Here's how the part is built. I have some questions about the finished solid (model axes, mm). Face numbers are marked on the shaded views. Coordinates: 2 decimals unless noted, no trailing zeros. Write each loop counter-clockwise with the first axis right and the second up, starting at its lowest first coordinate (ties: lowest second). Pieces come first, ordered by that corner, then holes.
Item 1: I want a section at D-D (x = 6.5). Please give me the cut outline in (y, z).
Item 2: I want a section at B-B (z = 1). Please give me the cut outline in (x, y), and give its area (3 significant figures).
Item 3: I'm going to push flat-ended pins straight in: P1, Ø6.5, axis at y = 54.3, z = 7.5, coming from the -X side; P2, Ø7.5, axis at y = 50, z = 11, coming from the +X side; P3, Ø1.5, axis at x = 2, z = 10.5, coming from the +Y side; P4, Ø5, axis at x = -1, z = 9, coming from the -Y side. Where does each tip first touch, or does it pass through?
Item 4: I want a section at C-C (y = 37). Please give me the cut outline in (x, z), and give its area (3 significant figures).
Item 5: If we mould it in two halves opening along X, with no side actions, what happens to the marked faces 1, 2, 3 and 4? For each: pulls with the +X half, pulls with the -X half, needs draft (parallel to the pull), parting line crosses it, or undercut.
Item 6: I want a section at A-A (y = 2). Please give me the cut outline in (x, z), and give its area (3 significant figures).
Item 7: Please list where these lines run through material, in increasing order: line 1 (X direction, y = 49, z = 6.25); line 2 (X direction, y = 21, z = 7.5); line 3 (Y direction, x = -5.75, z = 5.75).
from build123d import *

# Parameters (mm, degrees)
F1_DEPTH       = 15
F3_D           = 5.2
F3_DEPTH       = 30
F3_CBORE_D     = 10.2
F3_CBORE_DEPTH = 5
F3_TIP         = 1.5622376095
F4_W           = 8.2
F4_H           = 4.3
F5_DEPTH       = 12.4
F6_R           = 4.1
F7_DEPTH       = 25
F8_R           = 7.5
F9_R           = 7.5
F10_R          = 7.49999
F11_SIZE       = 11
F12_T1_DEPTH   = 2.7
F12_T3_DEPTH   = 2.7
F12_T5_DEPTH   = 30.9885128676
F12_T10_DEPTH  = 59.2770257353
F12_T15_DEPTH  = 59.2770257353
F12_T21_DEPTH  = 59.2770257353
F12_T26_DEPTH  = 59.2770257353
F12_T32_DEPTH  = 59.2770257353
F12_T38_DEPTH  = 59.2770257353
F13_R          = 5


# Not quite as in the source:
# - a fillet or chamfer that OpenCascade refuses, or shapes differently, is made with other operations: its cross-section is extruded or revolved along the edge and cut away or added
# - a fillet or chamfer is up to 0.001 mm smaller than in the source, because OpenCascade refuses the exact size


with BuildPart() as f1:
    # F0 (on Top) → F1 (new body)
    with BuildSketch(Plane.XY):
        Polygon((-7.0407824647, 62.3018580846), (-7.0407824647, -7.6981419154), (7.9592175353, -7.6981419154), (7.9592175353, 46.3018580846), (5.2592175353, 46.3018580846), (5.2592175353, 62.3018580846), (2.9592175353, 62.3018580846), (2.9592175353, 46.3018580846), (0.2592175353, 46.3018580846), (0.2592175353, 62.3018580846), (-2.0407824647, 62.3018580846), (-2.0407824647, 46.3018580846), (-4.7407824647, 46.3018580846), (-4.7407824647, 62.3018580846), align=None)
    extrude(amount=F1_DEPTH)

    # F3
    with Locations(Plane.XZ.offset(7.6981419154)):
        with Locations((0.4592175353, 7.5)):
            CounterBoreHole(F3_D / 2, F3_CBORE_D / 2, F3_CBORE_DEPTH, depth=F3_DEPTH)
            with Locations((0, 0, -(F3_DEPTH + F3_TIP / 2))):  # 118° drill point
                Cone(0, F3_D / 2, F3_TIP, mode=Mode.SUBTRACT)

    # F4 (on face) → F5 (cut)
    with BuildSketch(Plane.XY.offset(15)):
        with Locations((0.4592175353, 14.4518580846)):
            Rectangle(F4_W, F4_H)
    extrude(amount=-F5_DEPTH, mode=Mode.SUBTRACT)

    # F6 (on face) → F7 (cut)
    with BuildSketch(Plane.YZ.offset(5.2592175353)):
        with Locations((54.3018580846, 7.5)):
            Circle(F6_R)
    extrude(amount=-F7_DEPTH, mode=Mode.SUBTRACT)

    # F8
    f8_edges = [f1.edges().sort_by_distance(p)[0] for p in [
        (-5.890782, 62.301858, 0),
    ]]
    fillet(f8_edges, radius=F8_R)

    # F9
    f9_edges = [f1.edges().sort_by_distance(p)[0] for p in [
        (-0.890782, 62.301858, 0),
        (4.109218, 62.301858, 0),
    ]]
    fillet(f9_edges, radius=F9_R)

    # F10 (radius 7.5 in the source; OpenCascade refuses exactly that, so slightly less here)
    f10_edges = [f1.edges().sort_by_distance(p)[0] for p in [
        (-5.890782, 62.301858, 15),
        (-0.890782, 62.301858, 15),
        (4.109218, 62.301858, 15),
    ]]
    fillet(f10_edges, radius=F10_R)

    # F11
    f11_edges = [f1.edges().sort_by_distance(p)[0] for p in [
        (-3.390782, 46.301858, 15),
        (1.609218, 46.301858, 15),
        (6.609218, 46.301858, 15),
    ]]
    chamfer(f11_edges, length=F11_SIZE)

    # F12: chamfer of 11 on 3 edges, made by hand

    # F12_s2 → F12_t1 (cut)
    with BuildSketch(Plane.YZ.offset(-4.7407824647)):
        Polygon((46.3018580846, 11), (35.3018580846, 0), (46.3018580846, 0), align=None)
    extrude(amount=F12_T1_DEPTH, mode=Mode.SUBTRACT)

    # F12_s4 → F12_t3 (cut)
    with BuildSketch(Plane.YZ.offset(0.2592175353)):
        Polygon((35.3018580846, 0), (46.3018580846, 11), (46.3018580846, 0), align=None)
    extrude(amount=F12_T3_DEPTH, mode=Mode.SUBTRACT)

    # F12_s6 → F12_t5 (cut)
    with BuildSketch(Plane.YZ.offset(5.2592175353)):
        Polygon((35.3018580846, 0), (46.3018580846, 11), (46.3018580846, 0), align=None)
    extrude(amount=F12_T5_DEPTH, mode=Mode.SUBTRACT)


with BuildPart() as f12_tool8:
    # F12_s9 → F12_t10 (new body)
    with BuildSketch(Plane.YZ.offset(26.247730403)):
        Polygon((46.3018580846, 11), (35.3018580846, 0), (46.3018580846, 0), align=None)
    extrude(amount=-F12_T10_DEPTH)

    split(bisect_by=Plane.YZ.offset(5.2592175353), keep=Keep.TOP)


with BuildPart() as f1_1:
    add(f1.part)

    # F12_t7: cut F12_tool8
    add(f12_tool8.part, mode=Mode.SUBTRACT)


with BuildPart() as f12_tool13:
    # F12_s14 → F12_t15 (new body)
    with BuildSketch(Plane.YZ.offset(26.247730403)):
        Polygon((46.3018580846, 11), (35.3018580846, 0), (46.3018580846, 0), align=None)
    extrude(amount=-F12_T15_DEPTH)

    split(bisect_by=Plane.YZ.offset(0.2592175353), keep=Keep.TOP)

    split(bisect_by=Plane.YZ.offset(2.9592175353), keep=Keep.BOTTOM)


with BuildPart() as f1_2:
    add(f1_1.part)

    # F12_t12: cut F12_tool13
    add(f12_tool13.part, mode=Mode.SUBTRACT)


with BuildPart() as f12_tool19:
    # F12_s20 → F12_t21 (new body)
    with BuildSketch(Plane.YZ.offset(31.247730403)):
        Polygon((35.3018580846, 0), (46.3018580846, 11), (46.3018580846, 0), align=None)
    extrude(amount=-F12_T21_DEPTH)

    split(bisect_by=Plane.YZ.offset(5.2592175353), keep=Keep.TOP)


with BuildPart() as f1_3:
    add(f1_2.part)

    # F12_t18: cut F12_tool19
    add(f12_tool19.part, mode=Mode.SUBTRACT)


with BuildPart() as f12_tool24:
    # F12_s25 → F12_t26 (new body)
    with BuildSketch(Plane.YZ.offset(31.247730403)):
        Polygon((35.3018580846, 0), (46.3018580846, 11), (46.3018580846, 0), align=None)
    extrude(amount=-F12_T26_DEPTH)

    split(bisect_by=Plane.YZ.offset(-2.0407824647), keep=Keep.BOTTOM)

    split(bisect_by=Plane.YZ.offset(-4.7407824647), keep=Keep.TOP)


with BuildPart() as f1_4:
    add(f1_3.part)

    # F12_t23: cut F12_tool24
    add(f12_tool24.part, mode=Mode.SUBTRACT)


with BuildPart() as f12_tool30:
    # F12_s31 → F12_t32 (new body)
    with BuildSketch(Plane.YZ.offset(36.247730403)):
        Polygon((35.3018580846, 0), (46.3018580846, 11), (46.3018580846, 0), align=None)
    extrude(amount=-F12_T32_DEPTH)

    split(bisect_by=Plane.YZ.offset(0.2592175353), keep=Keep.TOP)

    split(bisect_by=Plane.YZ.offset(2.9592175353), keep=Keep.BOTTOM)


with BuildPart() as f1_5:
    add(f1_4.part)

    # F12_t29: cut F12_tool30
    add(f12_tool30.part, mode=Mode.SUBTRACT)


with BuildPart() as f12_tool36:
    # F12_s37 → F12_t38 (new body)
    with BuildSketch(Plane.YZ.offset(36.247730403)):
        Polygon((35.3018580846, 0), (46.3018580846, 11), (46.3018580846, 0), align=None)
    extrude(amount=-F12_T38_DEPTH)

    split(bisect_by=Plane.YZ.offset(-2.0407824647), keep=Keep.BOTTOM)

    split(bisect_by=Plane.YZ.offset(-4.7407824647), keep=Keep.TOP)


with BuildPart() as f1_6:
    add(f1_5.part)

    # F12_t35: cut F12_tool36
    add(f12_tool36.part, mode=Mode.SUBTRACT)

    # F13
    f13_edges = [f1_6.edges().sort_by_distance(p)[0] for p in [
        (1.609218, 42.801858, 7.5),
        (6.609218, 42.801858, 7.5),
        (-3.390782, 42.801858, 7.5),
    ]]
    fillet(f13_edges, radius=F13_R)


solid = f1_6.part
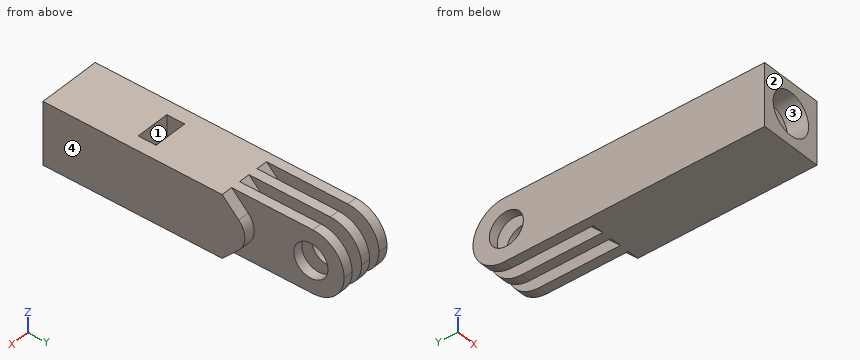
Answer:
1. outline: (-7.7, 0) - (35.3, 0) - (39.27, 3.96) arc R5 ccw to (39.27, 11.04) - (35.3, 15) - (-7.7, 15) - close
2. outline: (-7.04, -7.7) - (7.96, -7.7) - (7.96, 36.3) - (5.26, 36.3) - (5.26, 58.54) - (2.96, 58.54) - (2.96, 36.3) - (0.26, 36.3) - (0.26, 58.54) - (-2.04, 58.54) - (-2.04, 36.3) - (-4.74, 36.3) - (-4.74, 58.54) - (-7.04, 58.54) - close
2. area: 813 mm2
3. P1: passes through
3. P2: stops at x = 5.26
3. P3: stops at y = 40.2
3. P4: stops at y = -2.7
4. outline: (-7.04, 0) - (-4.74, 0) - (-4.74, 1.7) - (-2.04, 1.7) - (-2.04, 0) - (0.26, 0) - (0.26, 1.7) - (2.96, 1.7) - (2.96, 0) - (5.26, 0) - (5.26, 1.7) - (7.96, 1.7) - (7.96, 13.3) - (5.26, 13.3) - (5.26, 15) - (2.96, 15) - (2.96, 13.3) - (0.26, 13.3) - (0.26, 15) - (-2.04, 15) - (-2.04, 13.3) - (-4.74, 13.3) - (-4.74, 15) - (-7.04, 15) - close
4. area: 197 mm2
5. face 1: undercut
5. face 2: needs draft
5. face 3: undercut
5. face 4: pulls with the +X half
6. outline: (-7.04, 0) - (7.96, 0) - (7.96, 15) - (-7.04, 15) - close; hole circle Ø5.2 at (0.46, 7.5)
6. area: 204 mm2
7. line 1: x = -7.04 to -4.74, -2.04 to 0.26, 2.96 to 5.26
7. line 2: x = -7.04 to -2.14, 3.06 to 7.96
7. line 3: y = -7.7 to 50.59, 58.01 to 62.09
